Answer from the drawing. Dimensions are ordinates in mm from the lowest x, y and z of the part. Round coordinates to 2 decimals unless told otherwise and drop trailing zeros. Write each loop counter-clockwise with the first axis right and the second up, starting at its lowest first coordinate (ties: lowest second). Pieces come first, ordered by that corner, then holes. Notation, with made-up numbers: (74.25, -26.75) - (90.25, -26.75) arc R23 cw to (90.25, -10.75) - close; hole circle Ø4 at (23, 47). An arc over 180 degrees is marked (long way). Use a Markdown table: item, result. Add a question column.
1) Find the intervals of material crossed by probe 1 along Y at (x, z) = (11.3, 134); probe 2 along Y at (x, z) = (2, 60); probe 3 along Z at (x, y) = (3.25, 14), in increasing order. Write a range as from..to.
2) A cutting plane is placed at A-A (z = 134). Give the vertices of the cut face in (x, y).
3) Each of these flat-tipped pins is pushed along its axis until it touches: P1, Ø3, axis at y = 7.5, z = 31, coming from the +X side; P2, Ø12, axis at x = 6.5, z = 120.5, coming from the +Y side; P3, Ø1.5, axis at x = 10.5, z = 130, coming from the -Y side. Where does it stop, or does it pass through?
4) Determine the mould class of the marked faces 1 and 2 for opening direction Z: +Z half, -Z half, draft (parallel to the pull), parting line (faces both ways), or undercut.
5) A cutting plane is placed at C-C (x = 10). Give the vertices of the cut face in (y, z).
6) A cutting plane is placed at B-B (y = 10). Give the vertices of the cut face in (x, z), then the cut area to 3 significant figures.
7) A cutting plane is placed at D-D (z = 68). Give the vertices of the cut face in (x, y), then the cut area to 3 significant figures.
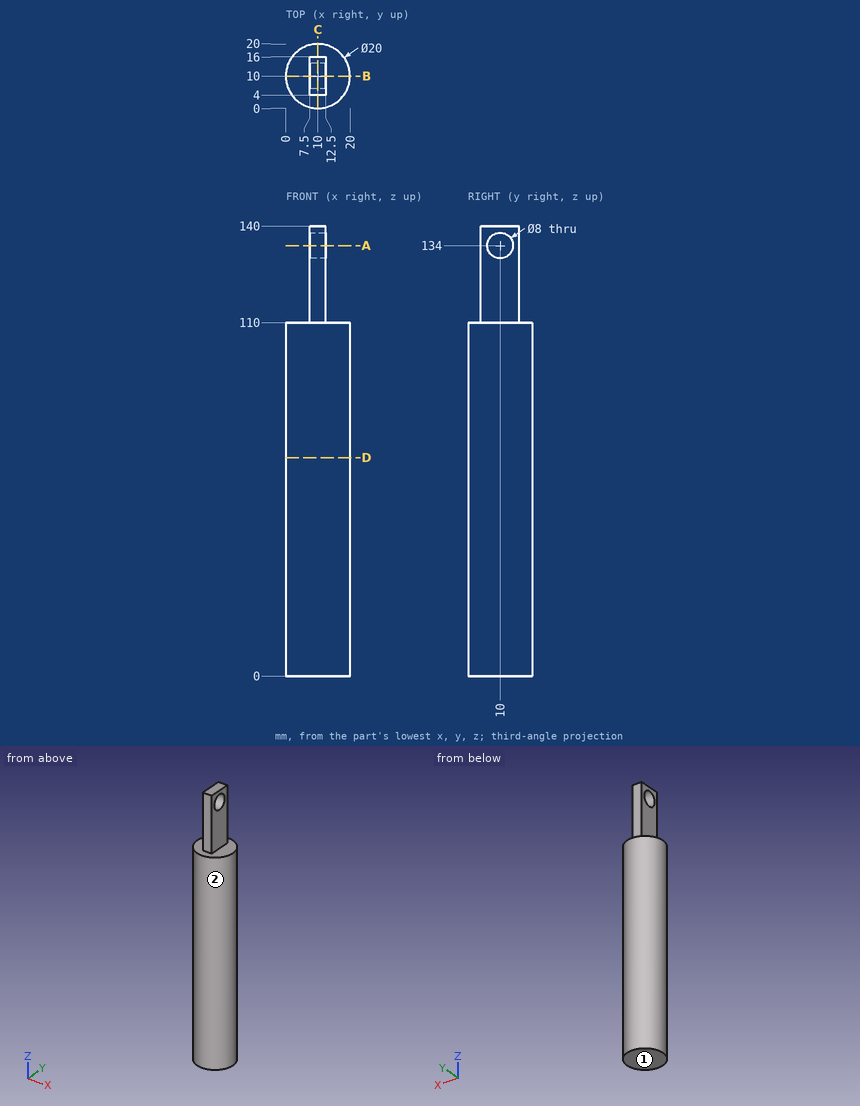
Entries:
| question | item | result |
|---|---|---|
| 1 | probe 1 | y = 4..6, 14..16 |
| 1 | probe 2 | y = 4..16 |
| 1 | probe 3 | z = 0..110 |
| 2 | outline | (7.5, 4) - (12.5, 4) - (12.5, 6) - (7.5, 6) - close; (7.5, 14) - (12.5, 14) - (12.5, 16) - (7.5, 16) - close |
| 3 | P1 | stops at x = 19.95 |
| 3 | P2 | stops at y = 16 |
| 3 | P3 | stops at y = 4 |
| 4 | face 1 | -Z half |
| 4 | face 2 | draft |
| 5 | outline | (0, 0) - (20, 0) - (20, 110) - (16, 110) - (16, 140) - (4, 140) - (4, 110) - (0, 110) - close; hole circle Ø8 at (10, 134) |
| 6 | outline | (0, 0) - (20, 0) - (20, 110) - (12.5, 110) - (12.5, 130) - (7.5, 130) - (7.5, 110) - (0, 110) - close; (7.5, 138) - (12.5, 138) - (12.5, 140) - (7.5, 140) - close |
| 6 | area | 2,310 mm² |
| 7 | outline | circle Ø20 at (10, 10) |
| 7 | area | 314 mm² |
